```python
from build123d import *

# Parameters (mm, degrees)
SKETCH_1_W        = 323
SKETCH_1_H        = 1020
EXTRUDE_1_DEPTH   = 25
SKETCH_3_W        = 323
SKETCH_3_H        = 980
EXTRUDE_2_DEPTH   = 25
SKETCH_15_W       = 283
SKETCH_15_H       = 920
EXTRUDE3_DEPTH    = 219
SKETCH3_W         = 323
SKETCH3_H         = 90
SKETCH3_R         = 9
SKETCH3_W_2       = 34
SKETCH3_H_2       = 50
EXTRUDE6_DEPTH    = 5
SKETCH4_W         = 34
SKETCH4_H         = 105
EXTRUDE7_DEPTH    = 10
SKETCH5_R         = 15
EXTRUDE8_DEPTH    = 76
SKETCH_17_R       = 28.5
EXTRUDE_1_2_DEPTH = 76
SKETCH_18_R       = 80
EXTRUDE_2_2_DEPTH = 20
SKETCH_19_R       = 28.5
EXTRUDE_3_DEPTH   = 90
SKETCH_20_R       = 80
EXTRUDE_4_DEPTH   = 20


with BuildPart() as part:
    # Эскиз1 → Extrude 1 (new body)
    with BuildSketch(Plane.XY):
        Rectangle(SKETCH_1_W, SKETCH_1_H)
    extrude(amount=EXTRUDE_1_DEPTH)



with BuildPart() as body_2:
    # Эскиз3 → Extrude 2 (new body)
    with BuildSketch(Plane(origin=(0, 0, -219), x_dir=(-1, 0, 0), z_dir=(0, 0, -1))):
        with Locations((0, 20)):
            Rectangle(SKETCH_3_W, SKETCH_3_H)
    extrude(amount=EXTRUDE_2_DEPTH)


with BuildPart() as part_1:
    add(part.part)

    add(body_2.part)  # Extrude3 merges body 2
    # Эскиз15 → Extrude3 (add)
    with BuildSketch(Plane(origin=(0, 0, 0), x_dir=(-1, 0, 0), z_dir=(0, 0, -1))):
        Rectangle(SKETCH_15_W, SKETCH_15_H)
    extrude(amount=EXTRUDE3_DEPTH)

    # Sketch3 → Extrude6 (add)
    # profile 1 of 2: a face of its own
    with BuildSketch(Plane.XZ.offset(510)):
        with Locations((0, 70)):
            Rectangle(SKETCH3_W, SKETCH3_H)
        with Locations(Location((-135, 75, 0), (0, 0, 270))):
            Circle(SKETCH3_R, mode=Mode.SUBTRACT)
        with Locations(Location((135, 75, 0), (0, 0, 270))):
            Circle(SKETCH3_R, mode=Mode.SUBTRACT)
    # profile 2 of 2: a face of its own
    with BuildSketch(Plane.XZ.offset(510)):
        with Locations((0, -355)):
            Rectangle(SKETCH3_W_2, SKETCH3_H_2)
        with Locations(Location((0, -355, 0), (0, 0, 270))):
            Circle(SKETCH3_R, mode=Mode.SUBTRACT)
    extrude(amount=-EXTRUDE6_DEPTH)


with BuildPart() as extrude6_piece_1:
    # of the separate pieces the step leaves, piece 1, a body of its own (extrude6_pieces)
    add(part_1.part.solids().sort_by_distance((161.5, 510, -219))[0])



with BuildPart() as extrude6_piece_2:
    # of the separate pieces the step leaves, piece 2, a body of its own (extrude6_pieces)
    add(part_1.part.solids().sort_by_distance((-17, -510, -380))[0])

    # Sketch4 → Extrude7 (add)
    with BuildSketch(Plane.XY.offset(-330)):
        with Locations((0, -457.5)):
            Rectangle(SKETCH4_W, SKETCH4_H)
    extrude(amount=EXTRUDE7_DEPTH)


with BuildPart() as extrude6_piece_1_1:
    add(extrude6_piece_1.part)

    add(extrude6_piece_2.part)  # Extrude8 merges Extrude6 piece 2
    # Sketch5 → Extrude8 (add)
    with BuildSketch(Plane(origin=(0, 0, -244), x_dir=(-1, 0, 0), z_dir=(0, 0, -1))):
        with Locations(Location((0, -420, 0), (0, 0, 90))):
            Circle(SKETCH5_R)
        with Locations((0, 430)):
            Circle(SKETCH5_R)
    extrude(amount=EXTRUDE8_DEPTH)

    # Эскиз17 → Extrude 1 2 (add)
    with BuildSketch(Plane.XY.offset(25)):
        with Locations((-65, -350)):
            Circle(SKETCH_17_R)
        with Locations((65, -350)):
            Circle(SKETCH_17_R)
        with Locations((-65, 393)):
            Circle(SKETCH_17_R)
        with Locations((65, 393)):
            Circle(SKETCH_17_R)
    extrude(amount=EXTRUDE_1_2_DEPTH)

    # Эскиз18 → Extrude 2 2 (add)
    with BuildSketch(Plane.XY.offset(101)):
        with Locations((-65, 393)):
            Circle(SKETCH_18_R)
        with Locations((-65, -350)):
            Circle(SKETCH_18_R)
    extrude(amount=-EXTRUDE_2_2_DEPTH)

    # Эскиз19 → Бобышка-Вытянуть3 (add)
    with BuildSketch(Plane.XY.offset(101)):
        with Locations((65, 393)):
            Circle(SKETCH_19_R)
        with Locations((65, -350)):
            Circle(SKETCH_19_R)
    extrude(amount=EXTRUDE_3_DEPTH)

    # Эскиз20 → Бобышка-Вытянуть4 (add)
    with BuildSketch(Plane.XY.offset(191)):
        with Locations((65, 393)):
            Circle(SKETCH_20_R)
        with Locations((65, -350)):
            Circle(SKETCH_20_R)
    extrude(amount=-EXTRUDE_4_DEPTH)


solid = extrude6_piece_1_1.part
```
Build history of the part. All positions in model axes, mm. A direction names the side the tool comes from. Coordinates: 2 decimals unless noted, no trailing zeros. Order: outer loops, then holes, each group sorted by start corner. A loop starts at its lowest first (then second) coordinate and runs counter-clockwise, first axis right, second up.
Item 1: Saw through at A-A on y = -142. List the corners of the cut face in (x, z).
Filled in:
outline: (-161.5, -244) - (161.5, -244) - (161.5, -219) - (141.5, -219) - (141.5, 0) - (161.5, 0) - (161.5, 25) - (-161.5, 25) - (-161.5, 0) - (-141.5, 0) - (-141.5, -219) - (-161.5, -219) - close
Item 2: Mould opens along Y. For faces 1 (the flat face through (144, 95, -219)), 2 (the flat face through (64, -384, 171)), 3 (the flat face through (-2, 510, 12)) say: released by +Y, released by -Y, zero draft, split by the parting line, or undercut.
Filled in:
face 1: zero draft
face 2: undercut
face 3: released by +Y
Item 3: Drill centre lines: L1, parallel to X at y = -508.55, z = 75; L2, parallel to X at y = -508.25, z = -355; L3, parallel to Y at x = 64.5, z = -234. Where is each one in solid material? Low to high.
Filled in:
L1: x = -161.5 to -144, -126 to 126, 144 to 161.5
L2: x = -17 to -9, 9 to 17
L3: y = -470 to 510
Item 4: Tool access for faces 4 (the flat face through (0, -454, -330)), 5 (the flat face through (17, -466, -328)), 6 (the flat face through (2, 460, -108)), 7 (the cylindrical face through (-5.745, -406.144, -281.468)): list every direction of +Z, -Z, +X, -X, +Y, -Y with a clear straight run to the whole face (end or side of a thin tool).
Filled in:
face 4: -Z, +X, -X, +Y
face 5: -Z, +X, +Y, -Y
face 6: +X, -X, +Y
face 7: none
Item 5: Saw through at B-B on y = -295. List the corners of the cut face in (x, z).
Filled in:
outline: (-161.5, -244) - (161.5, -244) - (161.5, -219) - (141.5, -219) - (141.5, 0) - (161.5, 0) - (161.5, 25) - (-161.5, 25) - (-161.5, 0) - (-141.5, 0) - (-141.5, -219) - (-161.5, -219) - close; (-123.09, 81) - (-6.91, 81) - (-6.91, 101) - (-123.09, 101) - close; (6.91, 171) - (123.09, 171) - (123.09, 191) - (6.91, 191) - close
Item 6: Drop flat-ended pins along their axis: pin 1 Ø8 at (x, y) = (120, -389) entering from -Z; pin 2 Ø3 at (x, y) = (53.5, -266) entering from +Z; pin 3 Ø8 at (x, z) = (-0.5, -323) entering from +Y; pin 4 Ø16 at (x, z) = (135, 75) entering from +Y. Give the stop position or say it passes through.
Filled in:
pin 1: stops at z = -244
pin 2: stops at z = 25
pin 3: stops at y = 445
pin 4: passes through
Item 7: Saw through at D-D on y = 393. List the corners of the cut face in (x, z).
Filled in:
outline: (-161.5, -244) - (161.5, -244) - (161.5, -219) - (141.5, -219) - (141.5, 0) - (161.5, 0) - (161.5, 25) - (93.5, 25) - (93.5, 171) - (145, 171) - (145, 191) - (-15, 191) - (-15, 171) - (36.5, 171) - (36.5, 25) - (-36.5, 25) - (-36.5, 81) - (15, 81) - (15, 101) - (-145, 101) - (-145, 81) - (-93.5, 81) - (-93.5, 25) - (-161.5, 25) - (-161.5, 0) - (-141.5, 0) - (-141.5, -219) - (-161.5, -219) - close
Item 8: Saw through at C-C on z = -177. List the corners of the cut face in (x, y), then the cut area to 3 significant figures.
Filled in:
outline: (-141.5, -460) - (141.5, -460) - (141.5, 460) - (-141.5, 460) - close
area: 260,000 mm2
